Model file for the job. Use its own axes, mm. A direction names the side the tool comes from. Give positions to 0.01 mm unless a question says otherwise; leave off trailing zeros. Loops run counter-clockwise (first coordinate to the right, second up) from the corner with the lowest first, then second, coordinate; pieces in that order, holes last. Notation, with made-up numbers: (55, -40) -> (107, -40) arc R33 ccw to (107, -12) -> close; hole circle Ø2 at (66.25, -30). An arc over 180 degrees is marked (long way). Use CSV: the item, a comma, the result in double quotes. Start each with the question number.
(1) Cut at B-B on y = -9.75. Write the cut outline in (x, z) (3 decimals).
(2) Cut at D-D on y = 6.75. Write the cut outline in (x, z) (3 decimals), then the cut area to 3 significant figures.
(3) Flat gauge pins, fed straight in: pin 1 (3 mm diameter, centred on x = 6.5, y = -2, fed in from -Z); pin 2 (1.3 mm diameter, centred on x = -9, z = 3, fed in from +Y). Where does each tip first touch, or does it go through?
(4) Drill centre lines: probe 1 along X at (y, z) = (2.75, 3.4) (3 decimals); probe 2 along X at (y, z) = (-2.5, 0.45) (3 decimals); probe 3 along X at (y, z) = (11, 3.8). Where is each one in solid material? Low to high.
(5) Cut at A-A on y = -5.5. Write the cut outline in (x, z) (3 decimals).
(6) Cut at C-C on z = 2.4. Write the cut outline in (x, y) (3 decimals), then the cut area to 3 significant figures.
(7) 3-axis set-ups, long thin cutter, end or side, ignore diameter. For faces 1 (the flat face through (-2.146, -6, 2)), 2 (the flat face through (-6.096, 3, 2)), 3 (the flat face through (-0.2, 0.2, 0)): which of +Z, -Z, +X, -X, +Y, -Y reach the whole face in a straight line?
from build123d import *

# Parameters (mm, degrees)
SKETCH1_W           = 31.75
SKETCH1_H           = 25.4
BOSS_EXTRUDE1_DEPTH = 4.2926
FILLET1_R           = 2.54
SKETCH2_W           = 4.2926
SKETCH2_H           = 19.05
SKETCH2_H_2         = 12.7
CUT_EXTRUDE2_DEPTH  = 4.2926


with BuildPart() as part:
    # Sketch1 → Boss-Extrude1 (new body)
    with BuildSketch(Plane.XY):
        Rectangle(SKETCH1_W, SKETCH1_H)
    extrude(amount=BOSS_EXTRUDE1_DEPTH)

    # Fillet1
    fillet1_edges = [part.edges().sort_by_distance(p)[0] for p in [
        (15.875, -12.7, 2.1463),
        (-15.875, -12.7, 2.1463),
        (-15.875, 12.7, 2.1463),
        (15.875, 12.7, 2.1463),
    ]]
    fillet(fillet1_edges, radius=FILLET1_R)

    # Sketch2 → Cut-Extrude2 (cut)
    with BuildSketch(Plane.XY.offset(4.2926)):
        with Locations((-8.2423, 3.175)):
            Rectangle(SKETCH2_W, SKETCH2_H)
        with Locations((8.2423, 3.175)):
            Rectangle(SKETCH2_W, SKETCH2_H)
        with Locations((0, -6.35)):
            Rectangle(SKETCH2_W, SKETCH2_H_2)
    extrude(amount=-CUT_EXTRUDE2_DEPTH, mode=Mode.SUBTRACT)


solid = part.part
Check result:
1,outline,"(-15.875, 0) -> (-2.146, 0) -> (-2.146, 4.293) -> (-15.875, 4.293) -> close; (2.146, 0) -> (15.875, 0) -> (15.875, 4.293) -> (2.146, 4.293) -> close"
2,outline,"(-15.875, 0) -> (-10.389, 0) -> (-10.389, 4.293) -> (-15.875, 4.293) -> close; (-6.096, 0) -> (6.096, 0) -> (6.096, 4.293) -> (-6.096, 4.293) -> close; (10.389, 0) -> (15.875, 0) -> (15.875, 4.293) -> (10.389, 4.293) -> close"
2,area,"99.4 mm²"
3,pin 1,"z = 0"
3,pin 2,"y = -6.35"
4,probe 1,"-15.875 to -10.389, -6.096 to 6.096, 10.389 to 15.875"
4,probe 2,"-15.875 to -10.389, -6.096 to -2.146, 2.146 to 6.096, 10.389 to 15.875"
4,probe 3,"-15.73 to -10.39, -6.1 to 6.1, 10.39 to 15.73"
5,outline,"(-15.875, 0) -> (-10.389, 0) -> (-10.389, 4.293) -> (-15.875, 4.293) -> close; (-6.096, 0) -> (-2.146, 0) -> (-2.146, 4.293) -> (-6.096, 4.293) -> close; (2.146, 0) -> (6.096, 0) -> (6.096, 4.293) -> (2.146, 4.293) -> close; (10.389, 0) -> (15.875, 0) -> (15.875, 4.293) -> (10.389, 4.293) -> close"
6,outline,"(-15.875, -10.16) arc R2.54 ccw to (-13.335, -12.7) -> (-2.146, -12.7) -> (-2.146, 0) -> (2.146, 0) -> (2.146, -12.7) -> (13.335, -12.7) arc R2.54 ccw to (15.875, -10.16) -> (15.875, 10.16) arc R2.54 ccw to (13.335, 12.7) -> (10.389, 12.7) -> (10.389, -6.35) -> (6.096, -6.35) -> (6.096, 12.7) -> (-6.096, 12.7) -> (-6.096, -6.35) -> (-10.389, -6.35) -> (-10.389, 12.7) -> (-13.335, 12.7) arc R2.54 ccw to (-15.875, 10.16) -> close"
6,area,"583 mm²"
7,face 1,"+Z, -Z, -Y"
7,face 2,"+Z, -Z, +Y"
7,face 3,"-Z, +X, -X, +Y, -Y"
